from build123d import *

# Parameters (mm, degrees)
F1_DEPTH = 105
F2_R     = 12
F3_DEPTH = 0.05
F4_W     = 50
F4_H     = 30
F5_DEPTH = 0.01


# Not quite as in the source:
# - ends of sketch curves that miss each other by under 0.0002 mm in the source are joined


with BuildPart() as f1:
    # F0 (on Front) → F1 (new body, symmetric)
    with BuildSketch(Plane.XZ):
        with BuildLine():
            Line((2.4999997663, 3.0085625581), (2.4999997663, -30.5))
            ThreePointArc((2.4999997663, -30.5), (3.9644658603, -34.0355339059), (7.4999997663, -35.5))
            Line((7.4999997663, -35.5), (12.4999997663, -35.5))
            ThreePointArc((12.4999997663, -35.5), (13.9142133287, -34.9142135624), (14.4999997663, -33.5))
            Line((14.4999997663, -33.5), (14.4999997663, 22.4999994828))
            ThreePointArc((14.4999997663, 22.4999994828), (12.4539129776, 29.7872458033), (6.9137199183, 34.9444437777))
            ThreePointArc((6.9137199183, 34.9444437777), (5.8016169865, 35.3591259101), (4.6231056877, 35.4999993303))
            Line((4.6231056877, 35.4999993303), (3.4999997663, 35.4999993303))
            ThreePointArc((3.4999997663, 35.4999993303), (2.0857862039, 34.9142128927), (1.4999997663, 33.4999993303))
            Line((1.4999997663, 33.4999993303), (1.4999997663, 30.2459664828))
            ThreePointArc((1.4999997663, 30.2459664828), (1.7397477835, 29.4324771221), (2.3823530195, 28.8790310431))
            ThreePointArc((2.3823530195, 28.8790310431), (-0.5000000985, 15.4999997293), (-3.3823532363, 28.8790310342))
            ThreePointArc((-3.3823532363, 28.8790310342), (-2.7397478169, 29.4324771961), (-2.4999997997, 30.2459665567))
            Line((-2.4999997997, 30.2459665567), (-2.4999997997, 33.5))
            ThreePointArc((-2.4999997997, 33.5), (-3.0857862373, 34.9142132361), (-4.4999997997, 35.4999996738))
            Line((-4.4999997997, 35.4999996738), (-4.6231058319, 35.4999996738))
            ThreePointArc((-4.6231058319, 35.4999996738), (-5.8016171306, 35.3591262536), (-6.9137200625, 34.9444441212))
            ThreePointArc((-6.9137200625, 34.9444441212), (-14.4718653147, 21.6128794539), (-5.288282, 9.344303))
            Line((-5.288282, 9.344303), (-0.7898995061, 7.707025658))
            ThreePointArc((-0.7898995061, 7.707025658), (1.5957599911, 5.8764447351), (2.4999997663, 3.0085625581))
        make_face()
    extrude(amount=F1_DEPTH, both=True)

    # F2 (on face) → F3 (join)
    with BuildSketch(Plane(origin=(2.4999997663, 0, 0), x_dir=(0, -1, 0), z_dir=(-1, 0, 0))):
        with Locations((0, -11.5)):
            Circle(F2_R)
    extrude(amount=F3_DEPTH)

    # F4 (on face) → F5 (join)
    with BuildSketch(Plane.YZ.offset(14.4999997663)):
        with Locations((0, -17.5000005172)):
            Rectangle(F4_W, F4_H)
    extrude(amount=F5_DEPTH)


solid = f1.part
The listing builds one solid part. Answer for the finished solid, in the listing's coordinates (mm). A direction names the side the tool comes from. Coordinates: 2 decimals unless noted, no trailing zeros. Order: outer loops, then holes, each group sorted by start corner. A loop starts at its lowest first (then second) coordinate and runs counter-clockwise, first axis right, second up. Notation, with made-up numbers: (7.25, -2.75) -> (38.25, -2.75) arc R18 ccw to (38.25, 3.25) -> close; hole circle Ø3 at (-8, 34). An arc over 180 degrees is marked (long way). Answer in a Markdown table with one row per item. Add a question column.
Item 1: Find section A-A (y = -35). Write down the section's boundary in (x, z), then the cut area to 3 significant figures.
Item 2: Find the intervals of material crossed by L1, parallel to X at y = -47, z = 22.5; L2, parallel to Z at x = -3, y = -96; L3, parallel to Z at x = -6.5, y = 34, in increasing order. Write a range as from..to.
Item 3: Determine the mould class of faces 1 (the face through (12.509, -1.47, 29.695)), 2 (the face through (-0.234, -1.47, 15.505)), 3 (the face through (-14.484, -1.47, 21.84)), 4 (the face through (3.93, -1.47, -34)) for opening direction Z: +Z half, -Z half, draft (parallel to the pull), parting line (faces both ways), or undercut.
Item 4: Which of the six approach directions +Z, -Z, +X, -X, +Y, -Y give full straight-line access (tool end or side, diameter ignored) to faces 5 (the face through (2.45, 0, -11)), 6 (the face through (14.51, 0, -17))?
Item 5: Each of these flat-tipped pins is pushed along its axis until it touches: P1, Ø12, axis at y = -5, z = -7.5, coming from the -X side; P2, Ø12, axis at y = 19.5, z = -6, coming from the -X side; P3, Ø12, axis at y = -51, z = -14, coming from the +X side. Where does it stop, or does it pass through?
Result set:
| question | item | result |
|---|---|---|
| 1 | outline | (-6.91, 34.94) arc R14 ccw to (-5.29, 9.34) -> (-0.79, 7.71) arc R5 cw to (2.5, 3.01) -> (2.5, -30.5) arc R5 ccw to (7.5, -35.5) -> (12.5, -35.5) arc R2 ccw to (14.5, -33.5) -> (14.5, 22.5) arc R14 ccw to (6.91, 34.94) arc R5 ccw to (4.62, 35.5) -> (3.5, 35.5) arc R2 ccw to (1.5, 33.5) -> (1.5, 30.25) arc R1.5 ccw to (2.38, 28.88) arc R7 cw (long way) to (-3.38, 28.88) arc R1.5 ccw to (-2.5, 30.25) -> (-2.5, 33.5) arc R2 ccw to (-4.5, 35.5) -> (-4.62, 35.5) arc R5 ccw to start |
| 1 | area | 1,030 mm² |
| 2 | L1 | x = -14.5..-7.5, 6.5..14.5 |
| 2 | L2 | z = 8.51..15.96, 29.13..34.82 |
| 2 | L3 | z = 9.85..18.89, 26.11..35.13 |
| 3 | face 1 | +Z half |
| 3 | face 2 | undercut |
| 3 | face 3 | parting line |
| 3 | face 4 | -Z half |
| 4 | face 5 | -Z, -X, +Y, -Y |
| 4 | face 6 | +Z, -Z, +X, +Y, -Y |
| 5 | P1 | stops at x = 2.45 |
| 5 | P2 | stops at x = 2.5 |
| 5 | P3 | stops at x = 14.5 |
